Geometry check sheet. Reference: the model listing, model coordinates, mm. Give positions to 0.01 mm unless a question says otherwise; leave off trailing zeros. Order: outer loops, then holes, each group sorted by start corner. A loop starts at its lowest first (then second) coordinate and runs counter-clockwise, first axis right, second up.
Autodesk Inventor part; units mm, degrees
ref_plane "YZ Plane" through (0, 0, 0) normal (1, 0, 0) x (0, 1, 0)
ref_plane "XZ Plane" through (0, 0, 0) normal (0, 1, 0) x (-1, 0, 0)
ref_plane "XY Plane" through (0, 0, 0) normal (0, 0, 1) x (1, 0, 0)
ref_plane "Work Plane3" through (0, 0, 0) normal (0, 0, 1) x (1, 0, 0)
sketch "Sketch1" plane through (0, 0, 0) normal (0, 0, 1) x (1, 0, 0)
  line L0 (-25.4, -893.191) -> (-25.4, -866.775)
  line L1 (-25.4, -893.191) -> (-23.241, -895.35)
  line L2 (-2.159, -895.35) -> (-23.241, -895.35)
  line L3 (-2.159, -895.35) -> (0, -893.191)
  line L4 (0, -866.775) -> (0, -893.191)
  arc A0 (3.175, -863.6) -> (0, -866.775) centre (3.175, -866.775) ccw
  line L5 (29.591, -863.6) -> (3.175, -863.6)
  line L6 (29.591, -863.6) -> (31.75, -861.441)
  line L7 (31.75, -840.359) -> (31.75, -861.441)
  line L8 (31.75, -840.359) -> (29.591, -838.2)
  line L9 (-54.991, -838.2) -> (29.591, -838.2)
  line L10 (-54.991, -838.2) -> (-57.15, -840.359)
  line L11 (-57.15, -861.441) -> (-57.15, -840.359)
  line L12 (-57.15, -861.441) -> (-54.991, -863.6)
  line L13 (-28.575, -863.6) -> (-54.991, -863.6)
  arc A1 (-25.4, -866.775) -> (-28.575, -863.6) centre (-28.575, -866.775) ccw
  circle A2 centre (12.7, -850.9) radius 2.0701
  circle A3 centre (0, -850.9) radius 2.0701
  circle A4 centre (-25.4, -850.9) radius 2.0701
  circle A5 centre (-50.8, -850.9) radius 2.0701
  circle A6 centre (-12.7, -876.3) radius 2.0701
  circle A7 centre (-12.7, -863.6) radius 2.0701
  circle A8 centre (-38.1, -850.9) radius 2.0701
  circle A9 centre (-12.7, -850.9) radius 2.0701
  circle A10 centre (-12.7, -889) radius 2.0701
  circle A11 centre (25.4, -850.9) radius 2.0701
  line L14 (-25.4, -863.6) -> (-25.4, -1498.6) construction
  line L15 (107.95, -863.6) -> (-361.95, -863.6)
  line L16 (-254, -893.191) -> (-254, -866.775)
  line L17 (-254, -893.191) -> (-251.841, -895.35)
  line L18 (-230.759, -895.35) -> (-251.841, -895.35)
  line L19 (-230.759, -895.35) -> (-228.6, -893.191)
  line L20 (-228.6, -866.775) -> (-228.6, -893.191)
  arc A12 (-225.425, -863.6) -> (-228.6, -866.775) centre (-225.425, -866.775) ccw
  line L21 (-199.009, -863.6) -> (-225.425, -863.6)
  line L22 (-199.009, -863.6) -> (-196.85, -861.441)
  line L23 (-196.85, -840.359) -> (-196.85, -861.441)
  line L24 (-196.85, -840.359) -> (-199.009, -838.2)
  line L25 (-283.591, -838.2) -> (-199.009, -838.2)
  line L26 (-283.591, -838.2) -> (-285.75, -840.359)
  line L27 (-285.75, -861.441) -> (-285.75, -840.359)
  line L28 (-285.75, -861.441) -> (-283.591, -863.6)
  line L29 (-257.175, -863.6) -> (-283.591, -863.6)
  arc A13 (-254, -866.775) -> (-257.175, -863.6) centre (-257.175, -866.775) ccw
  circle A14 centre (-215.9, -850.9) radius 2.0701
  circle A15 centre (-228.6, -850.9) radius 2.0701
  circle A16 centre (-254, -850.9) radius 2.0701
  circle A17 centre (-279.4, -850.9) radius 2.0701
  circle A18 centre (-241.3, -876.3) radius 2.0701
  circle A19 centre (-241.3, -863.6) radius 2.0701
  circle A20 centre (-266.7, -850.9) radius 2.0701
  circle A21 centre (-241.3, -850.9) radius 2.0701
  circle A22 centre (-241.3, -889) radius 2.0701
  circle A23 centre (-203.2, -850.9) radius 2.0701
  line L30 (-228.6, -863.6) -> (-228.6, -1498.6)
  line L31 (-361.95, -1498.6) -> (107.95, -1498.6)
  line L32 (0, -1469.009) -> (0, -1495.425)
  line L33 (0, -1469.009) -> (-2.159, -1466.85)
  line L34 (-23.241, -1466.85) -> (-2.159, -1466.85)
  line L35 (-23.241, -1466.85) -> (-25.4, -1469.009)
  line L36 (-25.4, -1495.425) -> (-25.4, -1469.009)
  arc A24 (-28.575, -1498.6) -> (-25.4, -1495.425) centre (-28.575, -1495.425) ccw
  line L37 (-54.991, -1498.6) -> (-28.575, -1498.6)
  line L38 (-54.991, -1498.6) -> (-57.15, -1500.759)
  line L39 (-57.15, -1521.841) -> (-57.15, -1500.759)
  line L40 (-57.15, -1521.841) -> (-54.991, -1524)
  line L41 (29.591, -1524) -> (-54.991, -1524)
  line L42 (29.591, -1524) -> (31.75, -1521.841)
  line L43 (31.75, -1500.759) -> (31.75, -1521.841)
  line L44 (31.75, -1500.759) -> (29.591, -1498.6)
  line L45 (3.175, -1498.6) -> (29.591, -1498.6)
  arc A25 (0, -1495.425) -> (3.175, -1498.6) centre (3.175, -1495.425) ccw
  circle A26 centre (-38.1, -1511.3) radius 2.0701
  circle A27 centre (-25.4, -1511.3) radius 2.0701
  circle A28 centre (0, -1511.3) radius 2.0701
  circle A29 centre (25.4, -1511.3) radius 2.0701
  circle A30 centre (-12.7, -1485.9) radius 2.0701
  circle A31 centre (-12.7, -1498.6) radius 2.0701
  circle A32 centre (12.7, -1511.3) radius 2.0701
  circle A33 centre (-12.7, -1511.3) radius 2.0701
  circle A34 centre (-12.7, -1473.2) radius 2.0701
  circle A35 centre (-50.8, -1511.3) radius 2.0701
  line L46 (-228.6, -1469.009) -> (-228.6, -1495.425)
  line L47 (-228.6, -1469.009) -> (-230.759, -1466.85)
  line L48 (-251.841, -1466.85) -> (-230.759, -1466.85)
  line L49 (-251.841, -1466.85) -> (-254, -1469.009)
  line L50 (-254, -1495.425) -> (-254, -1469.009)
  arc A36 (-257.175, -1498.6) -> (-254, -1495.425) centre (-257.175, -1495.425) ccw
  line L51 (-283.591, -1498.6) -> (-257.175, -1498.6)
  line L52 (-283.591, -1498.6) -> (-285.75, -1500.759)
  line L53 (-285.75, -1521.841) -> (-285.75, -1500.759)
  line L54 (-285.75, -1521.841) -> (-283.591, -1524)
  line L55 (-199.009, -1524) -> (-283.591, -1524)
  line L56 (-199.009, -1524) -> (-196.85, -1521.841)
  line L57 (-196.85, -1500.759) -> (-196.85, -1521.841)
  line L58 (-196.85, -1500.759) -> (-199.009, -1498.6)
  line L59 (-225.425, -1498.6) -> (-199.009, -1498.6)
  arc A37 (-228.6, -1495.425) -> (-225.425, -1498.6) centre (-225.425, -1495.425) ccw
  circle A38 centre (-266.7, -1511.3) radius 2.0701
  circle A39 centre (-254, -1511.3) radius 2.0701
  circle A40 centre (-228.6, -1511.3) radius 2.0701
  circle A41 centre (-203.2, -1511.3) radius 2.0701
  circle A42 centre (-241.3, -1485.9) radius 2.0701
  circle A43 centre (-241.3, -1498.6) radius 2.0701
  circle A44 centre (-215.9, -1511.3) radius 2.0701
  circle A45 centre (-241.3, -1511.3) radius 2.0701
  circle A46 centre (-241.3, -1473.2) radius 2.0701
  circle A47 centre (-279.4, -1511.3) radius 2.0701
  circle A48 centre (-76.2, -850.9) radius 2.0701
  circle A49 centre (-101.6, -850.9) radius 2.0701
  circle A50 centre (-127, -850.9) radius 2.0701
  circle A51 centre (-152.4, -850.9) radius 2.0701
  circle A52 centre (-177.8, -850.9) radius 2.0701
  circle A53 centre (-76.2, -1511.3) radius 2.0701
  circle A54 centre (-101.6, -1511.3) radius 2.0701
  circle A55 centre (-127, -1511.3) radius 2.0701
  circle A56 centre (-152.4, -1511.3) radius 2.0701
  circle A57 centre (-177.8, -1511.3) radius 2.0701
  circle A58 centre (-241.3, -1155.7) radius 2.0701
  circle A59 centre (-241.3, -1181.1) radius 2.0701
  circle A60 centre (-241.3, -1206.5) radius 2.0701
  circle A61 centre (-12.7, -1181.1) radius 2.0701
  circle A62 centre (-12.7, -1206.5) radius 2.0701
  circle A63 centre (-12.7, -1155.7) radius 2.0701
  line L60 (-63.5, -863.6) -> (-63.5, -838.2)
  line L61 (-63.5, -838.2) -> (-190.5, -838.2)
  line L62 (-190.5, -838.2) -> (-190.5, -863.6)
  line L63 (-25.4, -901.7) -> (-25.4, -1143)
  line L64 (0, -1143) -> (0, -1219.2)
  line L65 (0, -1219.2) -> (-25.4, -1219.2)
  line L66 (0, -1143) -> (-25.4, -1143)
  line L67 (-25.4, -1219.2) -> (-25.4, -1460.5)
  circle A64 centre (-12.7, -1155.7) radius 2.3813
  circle A65 centre (-12.7, -1181.1) radius 2.3812
  circle A66 centre (-12.7, -1206.5) radius 2.3813
  line L68 (-25.4, -901.7) -> (-63.5, -863.6)
  line L69 (-12.7, -1181.1) -> (-241.3, -1181.1)
  line L70 (-127, -850.9) -> (-127, -1511.3)
  line L71 (-228.6, -901.7) -> (-228.6, -1143)
  line L72 (-254, -1143) -> (-254, -1219.2)
  line L73 (-254, -1219.2) -> (-228.6, -1219.2)
  line L74 (-254, -1143) -> (-228.6, -1143)
  line L75 (-228.6, -1219.2) -> (-228.6, -1460.5)
  circle A67 centre (-241.3, -1155.7) radius 2.3813
  circle A68 centre (-241.3, -1181.1) radius 2.3812
  circle A69 centre (-241.3, -1206.5) radius 2.3813
  line L76 (-228.6, -901.7) -> (-190.5, -863.6)
  circle A70 centre (-177.8, -850.9) radius 2.3813
  circle A71 centre (-152.4, -850.9) radius 2.3813
  circle A72 centre (-127, -850.9) radius 2.3813
  circle A73 centre (-101.6, -850.9) radius 2.3813
  circle A74 centre (-76.2, -850.9) radius 2.3813
  line L77 (-63.5, -1498.6) -> (-63.5, -1524)
  line L78 (-63.5, -1524) -> (-190.5, -1524)
  line L79 (-190.5, -1524) -> (-190.5, -1498.6)
  line L80 (-25.4, -1460.5) -> (-63.5, -1498.6)
  line L81 (-228.6, -1460.5) -> (-190.5, -1498.6)
  circle A75 centre (-177.8, -1511.3) radius 2.3813
  circle A76 centre (-152.4, -1511.3) radius 2.3813
  circle A77 centre (-127, -1511.3) radius 2.3813
  circle A78 centre (-101.6, -1511.3) radius 2.3813
  circle A79 centre (-76.2, -1511.3) radius 2.3813
  point P0 (0, 0)
  dimension "d0" = 6.35
  dimension "d1" = 6.35
  dimension "d2" = 25.4
  dimension "d3" = 6.35
  dimension "d4" = 6.35
  dimension "d5" = 25.4
  dimension "d6" = 12.7
  dimension "d7" = 12.7
  dimension "d8" = 4.7625
  dimension "d9" = 4.7625
  dimension "d10" = 4.7625
extrude "Extrusion1" add sketch "Sketch1" along normal blind 6.35 contours L68 L63 L66 L64 L65 L67 L80 L31 L70 L15 | L15 L62 L61 L60 | L70 L69 L30 L76 L15 | L70 L31 L81 L30 L69 | L30 L73 L72 L74 | L31 L77 L78 L79
equation "\"d9\" = d8"
equation "\"d10\" = d8"
properties part number "Test_Swerve_Center" material "PMMA Plastic"
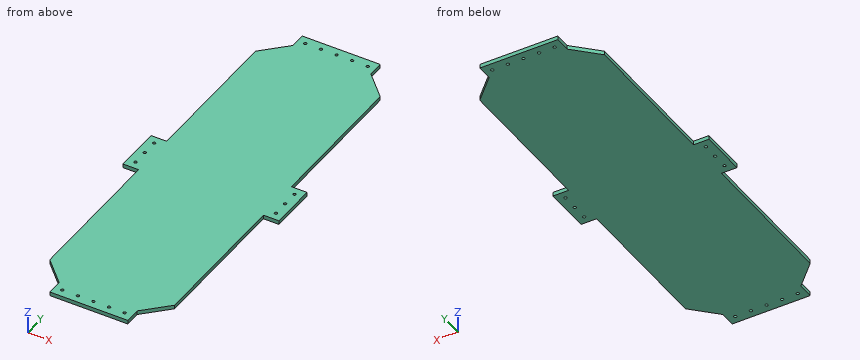
Item 1: Sectioned sample at B-B (z = 3.5). Give the number of separate pieces and of enclosed holes in the cut face, and give its area (3 significant figures).
Reported:
separate pieces: 1
enclosed holes: 16
area: 136,000 mm2
Item 2: Scan lines: L1, parallel to Y at x = -127, z = 3.75; L2, parallel to X at y = -850.9, z = 2; L3, parallel to Y at x = -12.7, z = 1.5. Record each from-to range of solid material in increasing order.
Reported:
L1: y = -1524 to -1513.68, -1508.92 to -853.28, -848.52 to -838.2
L2: x = -190.5 to -180.18, -175.42 to -154.78, -150.02 to -129.38, -124.62 to -103.98, -99.22 to -78.58, -73.82 to -63.5
L3: y = -1219.2 to -1208.88, -1204.12 to -1183.48, -1178.72 to -1158.08, -1153.32 to -1143
Item 3: Gauge pin test, flat ends, axial feed: pin 1 (4.5 mm diameter, centred on x = -127, y = -1511.3, fed in from +Z); pin 2 (3 mm diameter, centred on y = -846, z = 2.5, fed in from +X); pin 3 (3 mm diameter, centred on x = -240.5, z = 2.5, fed in from -Y); pin 4 (1.9 mm diameter, centred on y = -1069.5, z = 1.5, fed in from +X). Record the tip position at first contact, or that the pin passes through.
Reported:
pin 1: passes through
pin 2: stops at x = -63.5
pin 3: stops at y = -1219.2
pin 4: stops at x = -25.4
Item 4: Sectioned sample at C-C (y = -1376.5). Enter the section's corners in (x, z), and give its area (3 significant figures).
Reported:
outline: (-228.6, 0) - (-25.4, 0) - (-25.4, 6.35) - (-228.6, 6.35) - close
area: 1,290 mm2
Item 5: Sectioned sample at A-A (x = -221.5). Enter the section's corners in (y, z), and give its area (3 significant figures).
Reported:
outline: (-1467.6, 0) - (-894.6, 0) - (-894.6, 6.35) - (-1467.6, 6.35) - close
area: 3,640 mm2
